For this review, take the finished solid that the model builds, in its own axes (mm). A direction names the side the tool comes from. Coordinates: 2 decimals unless noted, no trailing zeros. Order: outer loops, then holes, each group sorted by start corner. A loop starts at its lowest first (then second) coordinate and runs counter-clockwise, first axis right, second up.
from build123d import *

# Parameters (mm, degrees)
SKETCH2_R                         = 31.732831761
CUT_EXTRUDE1_DEPTH                = 32.254845925
PIPE_TAP_DRILL_FOR_1_8_TAP1_D     = 8.4328
PIPE_TAP_DRILL_FOR_1_8_TAP1_DEPTH = 6.35
PIPE_TAP_DRILL_FOR_1_8_TAP1_TIP   = 2.533468714


with BuildPart() as part:
    # Sketch1 → Revolve1 (revolve)
    with BuildSketch(Plane(origin=(0, 0, 0), x_dir=(0, 0, -1), z_dir=(1, 0, 0)), mode=Mode.PRIVATE) as revolve1_sk:
        Polygon((3.175, 6.35), (3.175, 7.112), (6.35, 7.112), (6.35, 6.985), (7.62, 6.985), (7.62, 7.112), (10.795, 7.112), (10.795, 6.35), (13.97, 6.35), (13.97, 6.096), (19.05, 6.096), (19.05, 17.520886019), (31.75, 17.520886019), (31.75, 0), (12.7, 0), (12.7, 3.683), (0, 3.683), (0, 6.35), align=None)
    revolve(revolve1_sk.sketch.rotate(Axis((0, 0, -12.7), (0, 0, -1)), 180), axis=Axis((0, 0, -12.7), (0, 0, -1)))

    # Sketch2 → Cut-Extrude1 (cut, through all)
    with BuildSketch(Plane(origin=(0, 0, -19.05), x_dir=(-1, 0, 0), z_dir=(0, 0, -1))):
        Circle(SKETCH2_R)
        Polygon((7.332348419, 0), (3.666174209, 6.35), (-3.666174209, 6.35), (-7.332348419, 0), (-3.666174209, -6.35), (3.666174209, -6.35), align=None, mode=Mode.SUBTRACT)
    extrude(amount=CUT_EXTRUDE1_DEPTH, mode=Mode.SUBTRACT)

    # Pipe Tap Drill for 1/8 Tap1
    with Locations(Plane(origin=(0, 0, -31.75), x_dir=(-1, 0, 0), z_dir=(0, 0, -1))):
        with Locations((0, 0)):
            Hole(PIPE_TAP_DRILL_FOR_1_8_TAP1_D / 2, depth=PIPE_TAP_DRILL_FOR_1_8_TAP1_DEPTH)
            with Locations((0, 0, -(PIPE_TAP_DRILL_FOR_1_8_TAP1_DEPTH + PIPE_TAP_DRILL_FOR_1_8_TAP1_TIP / 2))):  # 118° drill point
                Cone(0, PIPE_TAP_DRILL_FOR_1_8_TAP1_D / 2, PIPE_TAP_DRILL_FOR_1_8_TAP1_TIP, mode=Mode.SUBTRACT)


solid = part.part
1. To check wall thickness, follow L1, parallel to X at y = 0, z = -8; L2, parallel to Y at x = 0, z = -29.25; L3, parallel to Z at x = 3.25, y = 6 (3 decimals). State the ranges of each line that lie inside material, in increasing order.
Answer below:
L1: x = -7.11 to -3.68, 3.68 to 7.11
L2: y = -6.35 to -4.22, 4.22 to 6.35
L3: z = -31.75 to -19.05, -10.795 to -3.175
2. Take a section at C-C, the plane x = -5.5. Give the boundary of the cut face in (y, z) (3 decimals), plus the area to 3 significant figures.
Answer below:
outline: (-4.509, -10.795) - (-3.174, -10.795) - (-3.174, -13.97) - (-2.629, -13.97) - (-2.629, -19.05) - (-3.174, -19.05) - (-3.174, -31.75) - (3.174, -31.75) - (3.174, -19.05) - (2.629, -19.05) - (2.629, -13.97) - (3.174, -13.97) - (3.174, -10.795) - (4.509, -10.795) - (4.509, -7.62) - (4.306, -7.62) - (4.306, -6.35) - (4.509, -6.35) - (4.509, -3.175) - (3.174, -3.175) - (3.174, 0) - (-3.174, 0) - (-3.174, -3.175) - (-4.509, -3.175) - (-4.509, -6.35) - (-4.306, -6.35) - (-4.306, -7.62) - (-4.509, -7.62) - close
area: 216 mm2
3. Clearance check with flat-ended pins moving along their axes: pin 1 Ø5 at (y, z) = (-5, -7.5) entering from -X; pin 2 Ø5 at (x, z) = (-2, -24) entering from -Y; pin 3 Ø1 at (x, z) = (-2.5, -18) entering from +Y. State where each tip first meets the part, or that it passes through.
Answer below:
pin 1: stops at x = -6.66
pin 2: stops at y = -6.35
pin 3: stops at y = 5.76
4. Take a section at A-A, the plane z = -3.5. Give the boundary of the cut face in (x, y), plus the area to 3 significant figures.
Answer below:
outline: circle Ø14.22 at (0, 0); hole circle Ø7.37 at (0, 0)
area: 116 mm2
5. Machinability: for faces 1 (the face through (3, 3, 0)), 2 (the face through (5.634, -2.93, -1.61)), 3 (the face through (-6, 3, -10.795)), 4 (the face through (-5.525, 3.131, -25.311)), 5 (the face through (-5.474, -3.219, -25.311)), which of the approach directions +Z, -Z, +X, -X, +Y, -Y give a long, thin tool a straight path to every point of the face, cutting with its end or side? Answer none if there is none.
Answer below:
face 1: +Z, +X, -X, +Y, -Y
face 2: +Z
face 3: none
face 4: -Z, -X, +Y
face 5: -Z, -X, -Y
6. The part is to be moulded in two halves that separate along Z. For faces 6 (the face through (5.525, -3.131, -25.311)), 7 (the face through (2, 4, -31.75)), 8 (the face through (-6.044, 0.794, -16.546)), say which applies: +Z half, -Z half, draft (parallel to the pull), parting line (faces both ways), or undercut.
Answer below:
face 6: draft
face 7: -Z half
face 8: undercut
7. Take a section at B-B, the plane z = -22. Give the boundary of the cut face in (x, y), plus the area to 3 significant figures.
Answer below:
outline: (-7.33, 0) - (-3.67, -6.35) - (3.67, -6.35) - (7.33, 0) - (3.67, 6.35) - (-3.67, 6.35) - close
area: 140 mm2
